```python
from build123d import *

# Parameters (mm, degrees)
F0_W     = 25.4
F0_H     = 30.48
F0_R     = 4.191
F1_DEPTH = 12.7
F0_H_2   = 7.62
F2_DEPTH = 38.1
F4_D     = 8.382
F4_DEPTH = 12.7


with BuildPart() as f1:
    # F0 (on Front) → F1 (new body)
    with BuildSketch(Plane.XZ):
        with Locations((0, 3.81)):
            Rectangle(F0_W, F0_H)
        with Locations((0, 9.779)):
            Circle(F0_R, mode=Mode.SUBTRACT)
    extrude(amount=F1_DEPTH)

    # F0 (on Front) → F2 (join)
    with BuildSketch(Plane.XZ):
        with Locations((0, -15.24)):
            Rectangle(F0_W, F0_H_2)
    extrude(amount=F2_DEPTH)

    # F4
    with Locations(Plane.XY.offset(-11.43)):
        with Locations((0, -25.4)):
            Hole(F4_D / 2, depth=F4_DEPTH)


solid = f1.part
```
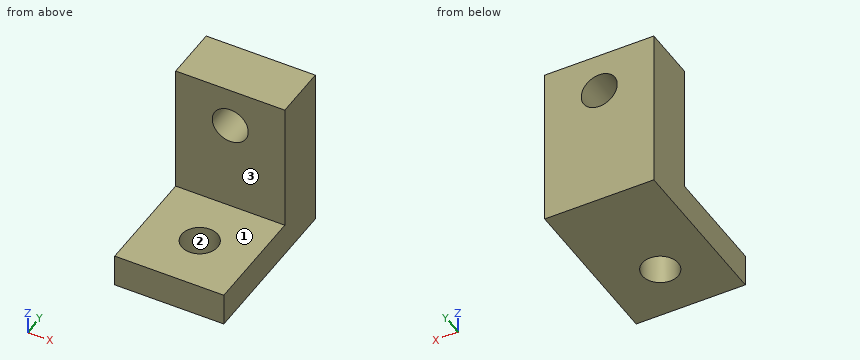
Verification items for the finished model (mm, model axes). Face numbers are marked on the shaded views. Give positions to 0.01 mm unless a question says otherwise; leave off trailing zeros. Order: outer loops, then holes, each group sorted by start corner. A loop starts at its lowest first (then second) coordinate and runs counter-clockwise, first axis right, second up. Notation, with made-up numbers: M 47.5,77.25 L 104.5,77.25 A21 ccw 104.5,84.25 Z; hole C 20,82 d2. An arc over 180 degrees is marked long. Answer in a Markdown table with one row per item. Add a question column.
Item 1: Scan lines: probe 1 along Y at (x, z) = (0, -14.25); probe 2 along Z at (x, y) = (0, -8.75); probe 3 along Z at (x, y) = (-8.5, -14). Record each from-to range of solid material in increasing order. Write a range as from..to.
Item 2: Section check A-A, the plane y = -25.4. Enter the section's corners in (x, z), and give its area (3 significant figures).
Item 3: Mould release check, pull along Y, two halves, no side actions. Record for the marked faces 1, 2 and 3: released by +Y, released by -Y, zero draft, split by the parting line, or undercut.
Item 4: Section check C-C, the plane x = -4.75. Enter the section's corners in (y, z), and give its area (3 significant figures).
Item 5: Section check B-B, the plane x = 0. Enter the section's corners in (y, z).
Item 6: Gauge pin test, flat ends, axial feed: pin 1 (6.5 mm diameter, centred on x = 0, y = -25.4, fed in from +Z); pin 2 (12 mm diameter, centred on x = 8.5, z = 10, fed in from -Y). Record the tip position at first contact, or that the pin passes through.
Item 7: Section check D-D, the plane y = -16. Enter the section's corners in (x, z), and give its area (3 significant figures).
Filled sheet:
| question | item | result |
|---|---|---|
| 1 | probe 1 | y = -38.1..-29.59, -21.21..0 |
| 1 | probe 2 | z = -19.05..5.59, 13.97..19.05 |
| 1 | probe 3 | z = -19.05..-11.43 |
| 2 | outline | M -12.7,-19.05 L -4.19,-19.05 L -4.19,-11.43 L -12.7,-11.43 Z; M 4.19,-19.05 L 12.7,-19.05 L 12.7,-11.43 L 4.19,-11.43 Z |
| 2 | area | 130 mm^2 |
| 3 | face 1 | zero draft |
| 3 | face 2 | undercut |
| 3 | face 3 | released by -Y |
| 4 | outline | M -38.1,-19.05 L 0,-19.05 L 0,19.05 L -12.7,19.05 L -12.7,-11.43 L -38.1,-11.43 Z |
| 4 | area | 677 mm^2 |
| 5 | outline | M -38.1,-19.05 L -29.59,-19.05 L -29.59,-11.43 L -38.1,-11.43 Z; M -21.21,-19.05 L 0,-19.05 L 0,5.59 L -12.7,5.59 L -12.7,-11.43 L -21.21,-11.43 Z; M -12.7,13.97 L 0,13.97 L 0,19.05 L -12.7,19.05 Z |
| 6 | pin 1 | passes through |
| 6 | pin 2 | stops at y = -12.7 |
| 7 | outline | M -12.7,-19.05 L 12.7,-19.05 L 12.7,-11.43 L -12.7,-11.43 Z |
| 7 | area | 194 mm^2 |
